CAD build for the part. Positions are in the model's coordinates, mm. A direction names the side the tool comes from. Round coordinates to 2 decimals unless told otherwise and drop trailing zeros. Loops run counter-clockwise (first coordinate to the right, second up) from the corner with the lowest first, then second, coordinate; pieces in that order, holes last.
```python
from build123d import *

# Parameters (mm, degrees)
PAD017_DEPTH           = 5
PAD020_DEPTH           = 6.25
SKETCH114_W            = 5.2
SKETCH114_H            = 1.65
PAD085_DEPTH           = 2.5
SKETCH115_W            = 5.2
SKETCH115_H            = 1.65
PAD086_DEPTH           = 5
LINEARPATTERN027_COUNT = 2
LINEARPATTERN027_PITCH = 3.3


with BuildPart() as obj1:
    # Sketch034 → Pad017 (new body)
    with BuildSketch(Plane.XY):
        with BuildLine():
            Line((-1.35, -1.8), (-1.35, 6))
            ThreePointArc((0, 7.35), (-0.954594, 6.954594), (-1.35, 6))
            Line((0, 9), (0, 7.35))
            Line((-2.6, 9), (0, 9))
            Line((-2.6, -1.8), (-2.6, 9))
            Line((-3.85, -1.8), (-2.6, -1.8))
            ThreePointArc((-3.85, -1.8), (-3.439949, -2.789949), (-2.45, -3.2))
            Line((-1.35, -3.2), (-2.45, -3.2))
            Line((-1.35, -1.8), (-1.35, -3.2))
        make_face()
    extrude(amount=PAD017_DEPTH)

    # Sketch037 → Pad020 (join)
    with BuildSketch(Plane.XY):
        Polygon((-1.35, 0.2), (-1.35, 1.6), (-2.6, 1.6), (-3.85, 1.6), (-3, 0.2), (-2.6, 0.2), align=None)
    extrude(amount=PAD020_DEPTH)


with BuildPart() as obj2:
    # Mirror001: instance of _obj1
    add(obj1.part.mirror(Plane(origin=(0, 0, 0), x_dir=(0, 1, 0), z_dir=(-1, 0, 0))))


with BuildPart() as body043:
    # Fusion001 base: copy of _obj1
    add(obj1.part)

    # Fusion001: union _obj2)
    add(obj2.part)

    # Sketch114 → Pad085 (new body)
    with BuildSketch(Plane.XY):
        with Locations((0, 9.825)):
            Rectangle(SKETCH114_W, SKETCH114_H)
    pad085 = extrude(amount=PAD085_DEPTH)

    # Sketch115 → Pad086 (join)
    with BuildSketch(Plane.XY):
        with Locations((0, 11.475)):
            Rectangle(SKETCH115_W, SKETCH115_H)
    pad086 = extrude(amount=PAD086_DEPTH)

    # LinearPattern027: Pad085, Pad086 ×2
    with Locations(*[(0, i * LINEARPATTERN027_PITCH, 0) for i in range(1, LINEARPATTERN027_COUNT)]):
        add(pad085)
        add(pad086)


solid = body043.part
```
Item 1: Cut at C-C, the plane x = 1. Give the cut face in (y, z), plus the area to 3 significant figures.
Answers follow:
outline: (6.91, 0) - (15.6, 0) - (15.6, 5) - (13.95, 5) - (13.95, 2.5) - (12.3, 2.5) - (12.3, 5) - (10.65, 5) - (10.65, 2.5) - (9, 2.5) - (9, 5) - (6.91, 5) - close
area: 35.2 mm2
Item 2: Two-plate mould, pull along X, no slides. Class faces 1 (the cylindrical face through (-3.45, -2.78, 2.46)), 2 (the flat face through (0, 10, 2.5)), 3 (the flat face through (-1.35, 1, 2)), 4 (the flat face through (3.43, 0.91, 3.08)): released by +X, released by -X, zero draft, split by the parting line, or undercut.
Answers follow:
face 1: released by -X
face 2: zero draft
face 3: undercut
face 4: released by +X
Item 3: Cut at D-D, the plane z = 2. Give the cut face in (x, y), plus the area to 3 significant figures.
Answers follow:
outline: (-3.85, -1.8) arc R1.4 ccw to (-2.45, -3.2) - (-1.35, -3.2) - (-1.35, 6) arc R1.35 cw to (0, 7.35) arc R1.35 cw to (1.35, 6) - (1.35, -3.2) - (2.45, -3.2) arc R1.4 ccw to (3.85, -1.8) - (2.6, -1.8) - (2.6, 0.2) - (3, 0.2) - (3.85, 1.6) - (2.6, 1.6) - (2.6, 15.6) - (-2.6, 15.6) - (-2.6, 1.6) - (-3.85, 1.6) - (-3, 0.2) - (-2.6, 0.2) - (-2.6, -1.8) - close
area: 75.0 mm2
Item 4: Probe line 1 (X direction, y = -1.25, z = 2); line 2 (Y direction, x = -1, z = 3.5); line 3 (X direction, y = 11, z = 2.5). List the from-to ranges inside material, lowest first.
Answers follow:
line 1: x = -2.6 to -1.35, 1.35 to 2.6
line 2: y = 6.91 to 9, 10.65 to 12.3, 13.95 to 15.6
line 3: x = -2.6 to 2.6
Item 5: Cut at A-A, the plane z = 5.5. Give the cut face in (x, y), plus the area to 3 significant figures.
Answers follow:
outline: (-3.85, 1.6) - (-3, 0.2) - (-1.35, 0.2) - (-1.35, 1.6) - close; (1.35, 0.2) - (3, 0.2) - (3.85, 1.6) - (1.35, 1.6) - close
area: 5.81 mm2
Item 6: 3-axis set-ups, long thin cutter, end or side, ignore diameter. For faces 5 (the flat face through (-2.6, 9, 2)), 6 (the flat face through (0, 12.3, 4)), 7 (the flat face through (0, 15, 5)), 8 (the flat face through (2.6, -1, 2)): which of +Z, -Z, +X, -X, +Y, -Y reach the whole face in a straight line?
Answers follow:
face 5: +Z, -Z, -X, +Y
face 6: +Z, +X, -X
face 7: +Z, +X, -X, +Y
face 8: +Z, -Z, +X
Item 7: Cut at B-B, the plane z = 4.25. State how many separate pieces and enclosed holes the cut face has, plus the area to 3 significant figures.
Answers follow:
separate pieces: 3
enclosed holes: 0
area: 57.9 mm2
Item 8: Flat gauge pins, fed straight in: P1, Ø2.5, axis at y = 9.5, z = 1.5, coming from the -X side; P2, Ø3, axis at x = -0.5, z = 4, coming from the -Y side; P3, Ø1.4, axis at x = -3.5, z = 1.5, coming from the +Y side; P4, Ø4, axis at x = -1, y = 5, coming from the +Z side. Where does each tip first touch, or does it go through?
Answers follow:
P1: stops at x = -2.6
P2: stops at y = -3.2
P3: stops at y = 1.6
P4: stops at z = 5
